from build123d import *

# Parameters (mm, degrees)
BOSS_EXTRUDE1_DEPTH      = 9
BOSS_EXTRUDE1_DEPTH_BACK = 9
SKETCH1_R                = 5.15
SKETCH2_R                = 2.5
BOSS_EXTRUDE2_DEPTH      = 5
BOSS_EXTRUDE3_START      = 5
SKETCH3_R                = 2.5
BOSS_EXTRUDE3_DEPTH      = 5
CHAMFER2_SIZE            = 0.5
FILLET1_R                = 0.2


with BuildPart() as part:
    # Sketch1 → Boss-Extrude1 (new, two sides: drawn at the far end of the back side and taken through both)
    with BuildSketch(Plane.XY.offset(-BOSS_EXTRUDE1_DEPTH_BACK)):
        Circle(SKETCH1_R)
    extrude(amount=BOSS_EXTRUDE1_DEPTH + BOSS_EXTRUDE1_DEPTH_BACK)

    # Sketch2 → Boss-Extrude2 (add)
    with BuildSketch(Plane.XY.offset(9)):
        Circle(SKETCH2_R)
    extrude(amount=BOSS_EXTRUDE2_DEPTH)

    # Sketch3 → Boss-Extrude3 (add)
    with BuildSketch(Plane(origin=(0, 0, -9), x_dir=(-1, 0, 0), z_dir=(0, 0, -1)).offset(BOSS_EXTRUDE3_START)):
        with Locations(Location((0, 0, 0), (0, 0, 180))):
            Circle(SKETCH3_R)
    extrude(amount=-BOSS_EXTRUDE3_DEPTH)

    # Chamfer2
    chamfer2_edges = [part.edges().sort_by_distance(p)[0] for p in [
        (-2.5, 0, -14),
        (-5.15, 0, 9),
        (-5.15, 0, -9),
        (-2.5, 0, 14),
    ]]
    chamfer(chamfer2_edges, length=CHAMFER2_SIZE)

    # Fillet1
    fillet1_edges = [part.edges().sort_by_distance(p)[0] for p in [
        (-2.5, 0, -9),
        (-2.5, 0, 9),
    ]]
    fillet(fillet1_edges, radius=FILLET1_R)


solid = part.part
Geometry check sheet. Reference: the model listing, model coordinates, mm. A direction names the side the tool comes from. Give positions to 0.01 mm unless a question says otherwise; leave off trailing zeros. Order: outer loops, then holes, each group sorted by start corner. A loop starts at its lowest first (then second) coordinate and runs counter-clockwise, first axis right, second up. Notation, with made-up numbers: (67, -14.5) - (99, -14.5) arc R9 ccw to (99, -0.5) - close; hole circle Ø3 at (-22.75, 84). An arc over 180 degrees is marked (long way). Use one line per item in the form item = value.
1) Depth check by flat-ended pin: pin 1 Ø1.5 at (x, z) = (4, 7) entering from -Y (3 decimals); pin 2 Ø2 at (y, z) = (1.5, 5) entering from -X; pin 3 Ø1.5 at (x, z) = (3, 11) entering from +Y; pin 4 Ø2 at (x, y) = (-1.5, -2) entering from -Z. Enter the tip coordinate at first touch or a pass-through.
Working result:
pin_1 = -3.995
pin_2 = -5.13
pin_3 = 1.09
pin_4 = -14
2) Access from +Z, -Z, +X, -X, +Y, -Y to the whole of each face (thin tool, end or side, straight path). Record for faces 1 (the face through (3, 0, -9)), 2 (the face through (-0.54, -2.44, 11.32)), 3 (the face through (0, 0, 14)).
Working result:
face_1 = -Z
face_2 = +Z
face_3 = +Z, +X, -X, +Y, -Y
3) Sectioned sample at D-D (z = -2.25). Record the boundary of the cut face in (x, y), and give its area (3 significant figures).
Working result:
outline = circle Ø10.3 at (0, 0)
area = 83.3 mm^2
4) Sectioned sample at A-A (x = 0). Record the boundary of the cut face in (y, z).
Working result:
outline = (-5.15, -8.5) - (-4.65, -9) - (-2.7, -9) arc R0.2 cw to (-2.5, -9.2) - (-2.5, -13.5) - (-2, -14) - (2, -14) - (2.5, -13.5) - (2.5, -9.2) arc R0.2 cw to (2.7, -9) - (4.65, -9) - (5.15, -8.5) - (5.15, 8.5) - (4.65, 9) - (2.7, 9) arc R0.2 cw to (2.5, 9.2) - (2.5, 13.5) - (2, 14) - (-2, 14) - (-2.5, 13.5) - (-2.5, 9.2) arc R0.2 cw to (-2.7, 9) - (-4.65, 9) - (-5.15, 8.5) - close
5) Sectioned sample at C-C (z = -10.5). Record the boundary of the cut face in (x, y).
Working result:
outline = circle Ø5 at (0, 0)
6) Material ranges on probe 1 along Z at (x, y) = (3.5, 2.75); probe 2 along Y at (x, z) = (-4.5, 0.5), recorded low to high. Write a range as from..to.
Working result:
probe_1 = -9..9
probe_2 = -2.5..2.5
